Autodesk Inventor part; units mm, degrees
ref_plane "YZ Plane" through (0, 0, 0) normal (1, 0, 0) x (0, 1, 0)
ref_plane "XZ Plane" through (0, 0, 0) normal (0, 1, 0) x (-1, 0, 0)
ref_plane "XY Plane" through (0, 0, 0) normal (0, 0, 1) x (1, 0, 0)
sketch "スケッチ1" plane through (0, 0, 0) normal (1, 0, 0) x (0, 1, 0)
  circle A0 centre (0, 0) radius 2
  line L0 (3.875, 0) -> (1.9375, 3.3558)
  line L1 (1.9375, 3.3558) -> (-1.9375, 3.3558)
  line L2 (-1.9375, 3.3558) -> (-3.875, 0)
  line L3 (-3.875, 0) -> (-1.9375, -3.3558)
  line L4 (-1.9375, -3.3558) -> (1.9375, -3.3558)
  line L5 (1.9375, -3.3558) -> (3.875, 0)
  dimension "d0" = 4
  dimension "d1" = 3.875
  dimension "d4" = 360
extrude "押し出し1" add sketch "スケッチ1" along normal blind 3.15
properties part number "4min-nut" material "アルミニウム 6061"
Geometry check sheet. Reference: the model listing, model coordinates, mm. Round coordinates to 2 decimals unless told otherwise and drop trailing zeros. Write each loop counter-clockwise with the first axis right and the second up, starting at its lowest first coordinate (ties: lowest second). Pieces come first, ordered by that corner, then holes. Notation, with made-up numbers: (-2.5, -29.5) -> (28.5, -29.5) arc R24 ccw to (28.5, -4.5) -> close; hole circle Ø3 at (32.5, -38.75). An arc over 180 degrees is marked (long way). One line per item, written item: value. Start each with the question number.
(1) Cross-section at C-C, the plane z = -0.5. Record the cut outline in (x, y).
(2) Scan lines: line 1 (Z direction, x = 1.5, y = 0); line 2 (Z direction, x = 1.4, y = -1.25); line 3 (Y direction, x = 2.3, z = 1). Record each from-to range of solid material in increasing order. Write a range as [from, to].
(3) Cross-section at A-A, the plane y = 0. Record the cut outline in (x, z), and give its area (3 significant figures).
(4) Cross-section at B-B, the plane x = 2.95. Record the cut outline in (y, z) (1 decimal), and give its area (3 significant figures).
(5) Draft check along Z on faces 1 (the cylindrical face through (2, 0, 2)), 2 (the flat face through (1.553, 2.893, -1.701)), 3 (the flat face through (3.15, 2, 2)). Enter one of: +Z half, -Z half, draft (parallel to the pull), parting line (faces both ways), or undercut.
(6) Go/stop test with flat-tipped pins: pin 1 Ø3.5 at (y, z) = (0, 0) entering from +X; pin 2 Ø1 at (x, y) = (2, -2.5) entering from +Z. Record where each tip stops, or that it passes through.
(7) Cross-section at D-D, the plane y = 3. Record the cut outline in (x, z).
Answer:
1. outline: (0, -3.59) -> (3.15, -3.59) -> (3.15, -1.94) -> (0, -1.94) -> close; (0, 1.94) -> (3.15, 1.94) -> (3.15, 3.59) -> (0, 3.59) -> close
2. line 1: [-3.36, -2], [2, 3.36]
2. line 2: [-3.36, -1.56], [1.56, 3.36]
2. line 3: [-3.3, -1.73], [1.73, 3.3]
3. outline: (0, -3.36) -> (3.15, -3.36) -> (3.15, -2) -> (0, -2) -> close; (0, 2) -> (3.15, 2) -> (3.15, 3.36) -> (0, 3.36) -> close
3. area: 8.54 mm²
4. outline: (-3.9, 0) -> (-1.9, -3.4) -> (1.9, -3.4) -> (3.9, 0) -> (1.9, 3.4) -> (-1.9, 3.4) -> close; hole circle Ø4 at (0, 0)
4. area: 26.4 mm²
5. face 1: undercut
5. face 2: -Z half
5. face 3: draft
6. pin 1: through
6. pin 2: z = 3.25
7. outline: (0, -1.52) -> (3.15, -1.52) -> (3.15, 1.52) -> (0, 1.52) -> close
